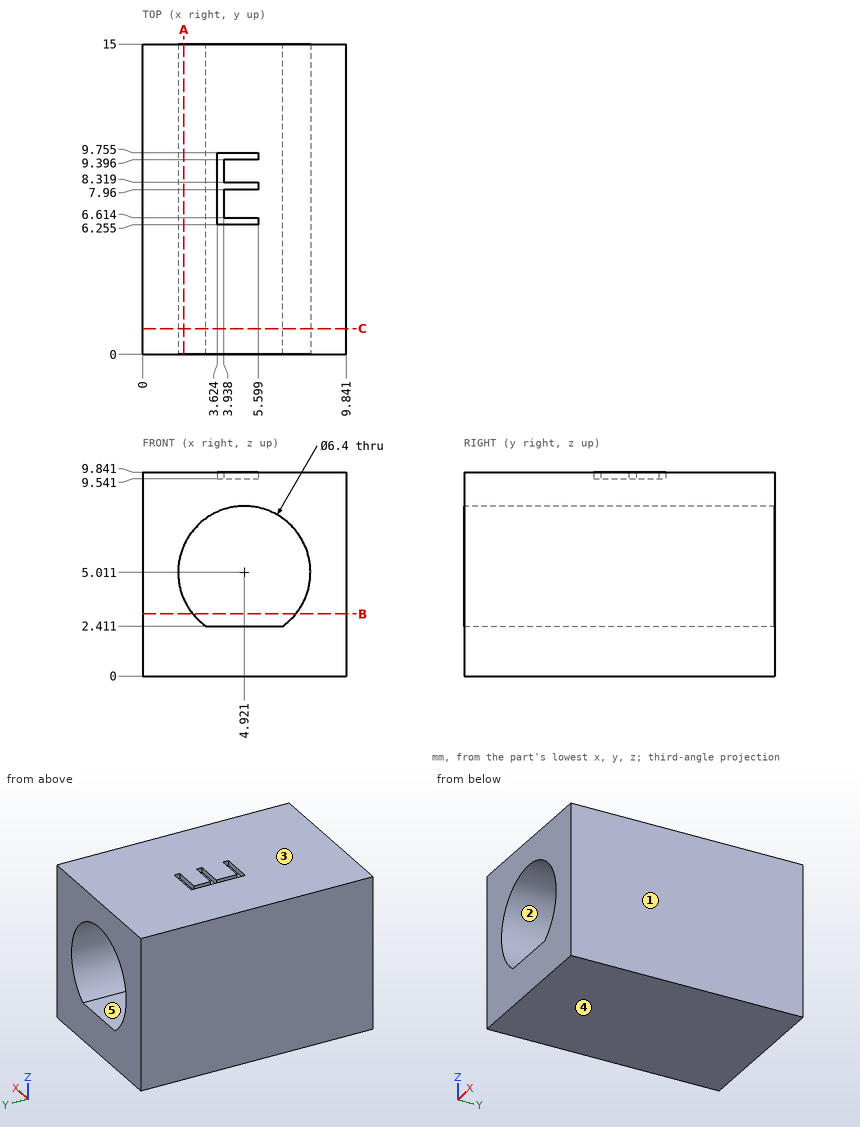
Verification items for this drawing (mm, ordinates from the low corner). A direction names the side the tool comes from. Give positions to 0.01 mm unless a question says otherwise; leave off trailing zeros. Write each loop counter-clockwise with the first axis right and the second up, starting at its lowest first coordinate (ties: lowest second). Pieces come first, ordered by that corner, then holes. Notation, with made-up numbers: (52.25, 72.5) -> (95.25, 72.5) arc R18 ccw to (95.25, 92.5) -> close; hole circle Ø7 at (-29, -25). An arc over 180 degrees is marked (long way). Write item = value, one per line.
Item 1: Gauge pin test, flat ends, axial feed: pin 1 (1.5 mm diameter, centred on x = 8, y = 7.5, fed in from -Z); pin 2 (2 mm diameter, centred on x = 6, z = 5, fed in from +Y). Record the tip position at first contact, or that the pin passes through.
Output:
pin_1 = 0
pin_2 = through
Item 2: Sectioned sample at C-C on y = 1.25. Record the boundary of the cut face in (x, z) (1 decimal).
Output:
outline = (0, 0) -> (9.8, 0) -> (9.8, 9.8) -> (0, 9.8) -> close; hole (3.1, 2.4) -> (6.8, 2.4) arc R3.2 ccw (long way) to start
Item 3: Sectioned sample at B-B on z = 3. Record the boundary of the cut face in (x, y).
Output:
outline = (0, 0) -> (2.43, 0) -> (2.43, 15) -> (0, 15) -> close; (7.41, 0) -> (9.84, 0) -> (9.84, 15) -> (7.41, 15) -> close
Item 4: Sectioned sample at A-A on x = 2. Record the boundary of the cut face in (y, z).
Output:
outline = (0, 0) -> (15, 0) -> (15, 3.7) -> (0, 3.7) -> close; (0, 6.32) -> (15, 6.32) -> (15, 9.84) -> (0, 9.84) -> close
Item 5: Release check for a two-part mould opening along X. For the marked faces 1, 2 and 3 record: +X half, -X half, draft (parallel to the pull), parting line (faces both ways), or undercut.
Output:
face_1 = +X half
face_2 = undercut
face_3 = draft
Item 6: Scan lines: probe 1 along Z at (x, y) = (4.75, 7); probe 2 along Z at (x, y) = (2, 1.5) (1 decimal); probe 3 along X at (y, z) = (14, 3.25). Record each from-to range of solid material in increasing order. Write a range as from..to.
Output:
probe_1 = 0..2.41, 8.21..9.84
probe_2 = 0..3.7, 6.3..9.8
probe_3 = 0..2.25, 7.59..9.84
Item 7: Tool access check on the marked faces 4 and 5. Record the directions out of +Z, -Z, +X, -X, +Y, -Y that give a thin tool (end or side, any length) a straight path to the whole face; none if there is none.
Output:
face_4 = -Z, +X, -X, +Y, -Y
face_5 = +Y, -Y
